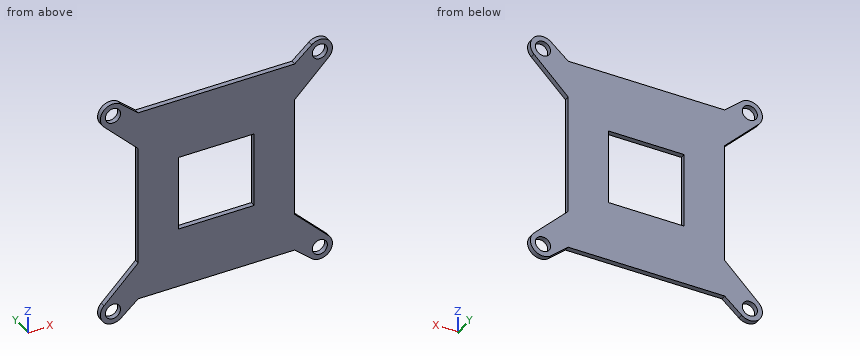
```python
from build123d import *

# Parameters (mm, degrees)
CROQUIS1_R              = 3
CROQUIS1_W              = 30
CROQUIS1_H              = 30
SALIENTE_EXTRUIR1_DEPTH = 2


with BuildPart() as part:
    # Croquis1 → Saliente-Extruir1 (new body)
    with BuildSketch(Plane(origin=(0, 0, 0), x_dir=(1, 0, 0), z_dir=(0, 1, 0))):
        with BuildLine():
            Line((-31, 39), (-37.741519768, 44.792401162))
            ThreePointArc((-37.741519768, 44.792401162), (-44.671057551, 44.394604021), (-44.526212448, 37.455169148))
            Line((-44.526212448, 37.455169148), (-31, 24))
            Line((-31, 24), (-31, -24))
            Line((-31, -24), (-44.526212448, -37.455169148))
            ThreePointArc((-44.526212448, -37.455169148), (-44.671057551, -44.394604021), (-37.741519768, -44.792401162))
            Line((-37.741519768, -44.792401162), (-31, -39))
            Line((-31, -39), (31, -39))
            Line((31, -39), (37.741519768, -44.792401162))
            ThreePointArc((37.741519768, -44.792401162), (44.671057551, -44.394604021), (44.526212448, -37.455169148))
            Line((44.526212448, -37.455169148), (31, -24))
            Line((31, -24), (31, 24))
            Line((31, 24), (44.526212448, 37.455169148))
            ThreePointArc((44.526212448, 37.455169148), (44.671057551, 44.394604021), (37.741519768, 44.792401162))
            Line((37.741519768, 44.792401162), (31, 39))
            Line((31, 39), (-31, 39))
        make_face()
        with Locations(Location((-41, 41, 0), (0, 0, 270))):
            Circle(CROQUIS1_R, mode=Mode.SUBTRACT)
        with Locations(Location((41, 41, 0), (0, 0, 270))):
            Circle(CROQUIS1_R, mode=Mode.SUBTRACT)
        with Locations(Location((41, -41, 0), (0, 0, 270))):
            Circle(CROQUIS1_R, mode=Mode.SUBTRACT)
        with Locations(Location((-41, -41, 0), (0, 0, 270))):
            Circle(CROQUIS1_R, mode=Mode.SUBTRACT)
        Rectangle(CROQUIS1_W, CROQUIS1_H, mode=Mode.SUBTRACT)
    extrude(amount=SALIENTE_EXTRUIR1_DEPTH)


solid = part.part
```
Could you check a few things on this model? Use its own coordinates, in mm. Coordinates: 2 decimals unless noted, no trailing zeros. Write each loop counter-clockwise with the first axis right and the second up, starting at its lowest first coordinate (ties: lowest second). Pieces come first, ordered by that corner, then holes. Notation, with made-up numbers: M 76,-13 L 103,-13 A19 ccw 103,16 Z; hole C 36,-10.75 d8. An arc over 180 degrees is marked long. Answer as CSV lines item,"result". Start each with the question number.
1) I want a section at D-D, the plane x = 41. Please give me the cut outline in (y, z).
2) I want a section at C-C, the plane z = -10.5. Please give me the cut outline in (x, y).
3) For P1, Ø1, axis at y = 1, z = 5, coming from the -X side; P2, Ø3.5, axis at x = -41, z = -41, coming from the +Y side; P3, Ø6, axis at x = 17, z = 28, coming from the -Y side; P4, Ø1, axis at x = 1.5, y = 1, coming from the +Z side, each with a flat end and sliding along its axis, tell me the tip position at first contact or that it passes through.
4) Please list where these lines run through material, in increasing order: line 1 (Z direction, x = -10, y = 1.8); line 2 (X direction, y = 1.35, z = 41); line 3 (Z direction, x = 39.5, y = 0.15). Write a range as from..to.
5) I want a section at A-A, the plane x = -9.5. Please give me the cut outline in (y, z), and give its area (3 significant figures).
6) I want a section at B-B, the plane y = 1.15. Please give me the cut outline in (x, z), and give its area (3 significant figures).
Data:
1,outline,"M 0,-46 L 2,-46 L 2,-44 L 0,-44 Z; M 0,-38 L 2,-38 L 2,-33.95 L 0,-33.95 Z; M 0,33.95 L 2,33.95 L 2,38 L 0,38 Z; M 0,44 L 2,44 L 2,46 L 0,46 Z"
2,outline,"M -31,0 L -15,0 L -15,2 L -31,2 Z; M 15,0 L 31,0 L 31,2 L 15,2 Z"
3,P1,"stops at x = -31"
3,P2,"passes through"
3,P3,"stops at y = 0"
3,P4,"stops at z = 39"
4,line 1,"z = -39..-15, 15..39"
4,line 2,"x = -46..-44, -38..-33.33, 33.33..38, 44..46"
4,line 3,"z = -45.77..-43.6, -38.4..-32.46, 32.46..38.4, 43.6..45.77"
5,outline,"M 0,-39 L 2,-39 L 2,-15 L 0,-15 Z; M 0,15 L 2,15 L 2,39 L 0,39 Z"
5,area,"96.0 mm^2"
6,outline,"M -44.53,-37.46 A5 ccw -37.74,-44.79 L -31,-39 L 31,-39 L 37.74,-44.79 A5 ccw 44.53,-37.46 L 31,-24 L 31,24 L 44.53,37.46 A5 ccw 37.74,44.79 L 31,39 L -31,39 L -37.74,44.79 A5 ccw -44.53,37.46 L -31,24 L -31,-24 Z; hole C -41,-41 d6; hole C -41,41 d6; hole M -15,-15 L 15,-15 L 15,15 L -15,15 Z; hole C 41,-41 d6; hole C 41,41 d6"
6,area,"4,560 mm^2"
